Autodesk Fusion 360 part; units mm, degrees
sketch "Sketch1" plane through (0, 0, 0) normal (0, 0, 1) x (1, 0, 0)
  line L0 (0, 0) -> (40, 0)
  line L1 (0, 0) -> (0, 85)
  line L2 (0, 85) -> (40, 85)
  line L3 (40, 85) -> (40, 0)
  line L4 (0, 0) -> (0, 5)
  line L5 (0, 5) -> (40, 5)
  line L6 (40, 5) -> (40, 0)
  line L7 (0, 5) -> (0, 20)
  line L8 (0, 20) -> (40, 20)
  line L9 (40, 20) -> (40, 5)
  line L10 (0, 85) -> (0, 70)
  line L11 (0, 70) -> (40, 70)
  line L12 (40, 70) -> (40, 85)
  line L13 (0, 70) -> (15, 70)
  line L14 (15, 70) -> (15, 20)
  line L15 (15, 20) -> (25, 20)
  line L16 (15, 20) -> (25, 20)
  line L17 (25, 20) -> (25, 70)
  line L18 (25, 70) -> (15, 70)
extrude "Extrude1" add sketch "Sketch1" along normal blind 25 contours L0 L1 L3 L4 L5 L6 makes body 1
extrude "Extrude2" add sketch "Sketch1" along normal blind 15 separate body contours L1 L8 L11 L13 L14 | L3 L8 L11 L17 makes body 2 at (0, 36.6667, 10) makes body 3 at (25, 36.6667, 10)
extrude "Extrude3" add sketch "Sketch1" along normal blind 20 contours L8 L11 L14 L15 L16 L17 L18 bodies 2 3
extrude "Extrude4" add sketch "Sketch1" along normal blind 25 contours L1 L2 L3 L10 L11 L12 L13 L18 bodies 2
extrude "Extrude5" add sketch "Sketch1" along normal blind 25 contours L1 L3 L5 L7 L8 L9 L15 L16 bodies 1 2
sketch "Sketch2" plane through (0, 0, 25) normal (0, 0, 1) x (-1, 0, 0)
  line L0 (0, 0) -> (-40, 0)
  line L1 (-40, 0) -> (-40, -20)
  line L2 (-40, -20) -> (0, -20)
  line L3 (0, -20) -> (0, 0)
  line L4 (0, -20) -> (0, -5)
  line L5 (-40, -5) -> (-40, -20)
  line L6 (0, -20) -> (-40, -20)
  line L7 (-40, -5) -> (0, -5)
sketch "Sketch3" plane through (40, 0, 0) normal (1, 0, 0) x (0, 1, 0)
  line L0 (0, 0) -> (85, 0)
  line L1 (85, 0) -> (85, 25)
  line L2 (85, 25) -> (70, 25)
  line L3 (70, 25) -> (70, 15)
  line L4 (70, 15) -> (20, 15)
  line L5 (20, 15) -> (20, 25)
  line L6 (20, 25) -> (0, 25)
  line L7 (0, 25) -> (0, 0)
  circle A0 centre (20, 25) radius 15
  line L8 (20, 25) -> (20, 40)
extrude "Extrude6" add sketch "Sketch3" against normal blind 40 contours L6 A0 L8 bodies 1
sketch "Sketch4" plane through (0, 85, 0) normal (0, 1, 0) x (-1, 0, 0)
  line L0 (-40, 0) -> (0, 0)
  line L1 (0, 0) -> (0, 25)
  line L2 (0, 25) -> (-40, 25)
  line L3 (-40, 25) -> (-40, 0)
  circle A0 centre (-20, 25) radius 10
  line L4 (-30, 25) -> (-10, 25)
extrude "Extrude7" add sketch "Sketch4" against normal blind 15 contours L2 A0 L4 picked at (-23.1513, 27.4288) bodies 1
sketch "Sketch5" plane through (0, 0, 0) normal (0, -1, 0) x (1, 0, 0)
  line L0 (0, 0) -> (40, 0)
  line L1 (40, 0) -> (40, 25)
  line L2 (40, 25) -> (0, 25)
  line L3 (0, 25) -> (0, 0)
  line L4 (0, 0) -> (10, 0)
  line L5 (10, 0) -> (10, 10)
  line L6 (10, 10) -> (15, 10)
  line L7 (15, 10) -> (15, 20)
  line L8 (15, 20) -> (25, 20)
  line L9 (25, 20) -> (25, 10)
  line L10 (25, 10) -> (30, 10)
  line L11 (30, 10) -> (30, 0)
  line L12 (30, 0) -> (10, 0)
sketch "Sketch6" plane through (0, 0, 0) normal (0, -1, 0) x (1, 0, 0)
extrude "Extrude8" cut sketch "Sketch5" against normal blind 20 contours L0 L5 L6 L7 L8 L9 L10 L11 L12 bodies 1
For this review, take the finished solid that the model builds, in its own axes (mm). A direction names the side the tool comes from. Coordinates: 2 decimals unless noted, no trailing zeros. Loops run counter-clockwise (first coordinate to the right, second up) from the corner with the lowest first, then second, coordinate; pieces in that order, holes last. Notation, with made-up numbers: (67.5, 29.5) -> (107.5, 29.5) arc R25 cw to (107.5, 50.5) -> close; hole circle Ø9 at (82, 64). An arc over 180 degrees is marked (long way). Return JSON: item names as keys, results as strings. Group by question number.
(1) To check wall thickness, follow L1, parallel to Y at x = 7.5, z = 21; L2, parallel to X at y = 19, z = 6; L3, parallel to Z at x = 17, y = 33. State the ranges of each line that lie inside material, in increasing order.
(2) Tool access review of faces 4 (the flat face through (27, 10, 10)), 5 (the cylindrical face through (20, 78, 35)), 6 (the flat face through (25, 45, 17)), 7 (the flat face through (20, 45, 20)): name each direction out of +Z, -Z, +X, -X, +Y, -Y from which nothing blocks a thin tool from reaching the whole face with its end or side.
(3) Consider section C-C, the plane y = 66. Give the boundary of the cut face in (x, z).
(4) Mouldability with a two-part tool opening along X and no side actions: class faces 1 (the flat face through (0, 42, 11)), 2 (the flat face through (20, 3, 25)), 3 (the flat face through (25, 10, 15)) as pulls with the +X half, pulls with the -X half, needs draft (parallel to the pull), parting line crosses it, or undercut.
(5) For pin 1 Ø3 at (y, z) = (13.5, 15) entering from -X; pin 2 Ø10 at (y, z) = (61, 20.5) entering from -X; pin 3 Ø5.5 at (x, y) = (27, 8) entering from -Z; pin 4 Ø11 at (x, y) = (21.5, 38.5) entering from +Z, all flat-tipped, find the tip position at first contact; note any pin that passes through.
(6) Consider section D-D, the plane x = 8.5. Give the boundary of the cut face in (y, z), plus the area to 3 significant figures.
Results below:
{
 "1": {"L1": "y = 0 to 20, 70 to 85", "L2": "x = 0 to 10, 30 to 40", "L3": "z = 0 to 20"},
 "2": {"face 4": "-Z, -Y", "face 5": "+Z, +Y", "face 6": "+Z, +X", "face 7": "+Z, +X, -X"},
 "3": {"outline": "(0, 0) -> (40, 0) -> (40, 15) -> (25, 15) -> (25, 20) -> (15, 20) -> (15, 15) -> (0, 15) -> close"},
 "4": {"face 1": "pulls with the -X half", "face 2": "needs draft", "face 3": "undercut"},
 "5": {"pin 1": "stops at x = 0", "pin 2": "stops at x = 15", "pin 3": "stops at z = 10", "pin 4": "stops at z = 20"},
 "6": {"outline": "(0, 0) -> (85, 0) -> (85, 25) -> (70, 25) -> (70, 15) -> (20, 15) -> (20, 40) arc R15 ccw to (5, 25) -> (0, 25) -> close", "area": "1,800 mm2"}
}
